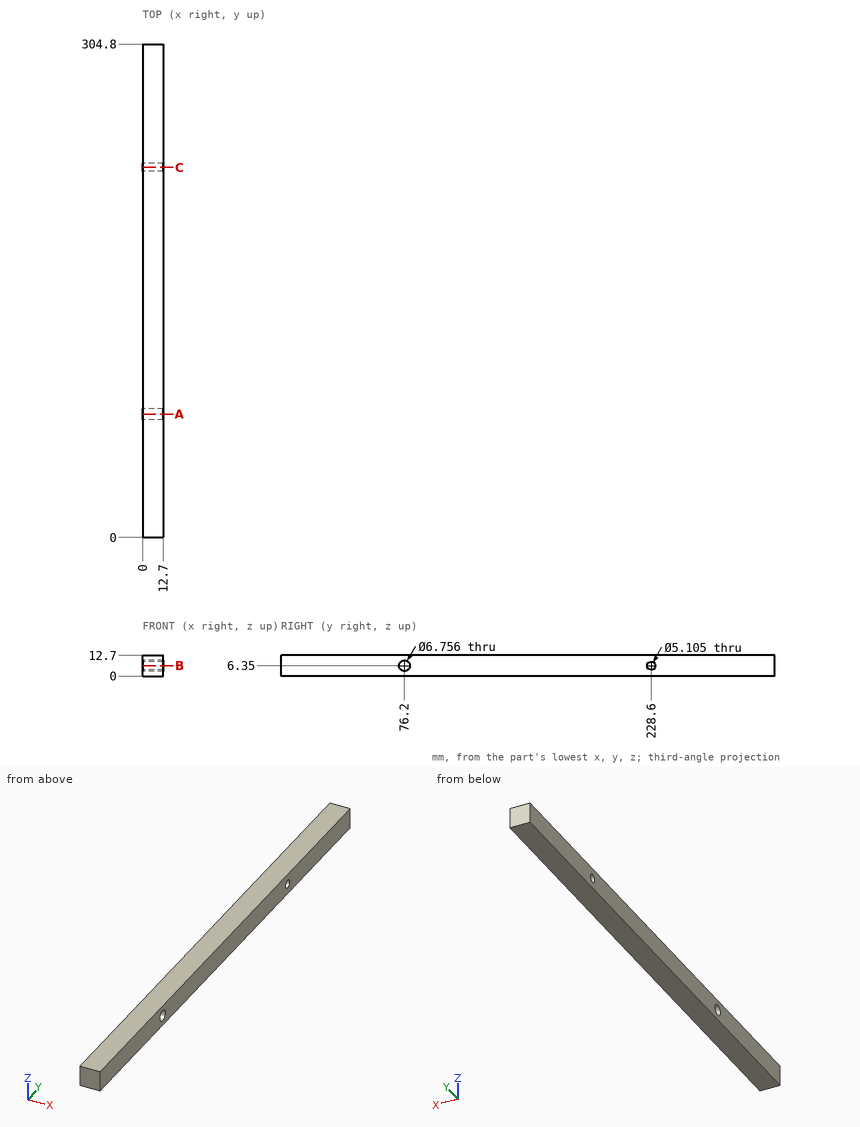
The drawing under review shows one solid part. Ordinate dimensions are in mm from its lowest x, y, z. Round coordinates to 2 decimals unless told otherwise and drop trailing zeros. Loops run counter-clockwise (first coordinate to the right, second up) from the corner with the lowest first, then second, coordinate; pieces in that order, holes last. Notation, with made-up numbers: (-6.75, 53.25) -> (3.25, 53.25) arc R30 cw to (3.25, 77.25) -> close; hole circle Ø7 at (82, 62). An arc over 180 degrees is marked (long way). Answer in a Markdown table with one row per item.
1) Consider section C-C, the plane y = 228.6. Write out the cut boundary in (x, z).
Taken from the geometry:
| item | result |
|---|---|
| outline | (0, 0) -> (12.7, 0) -> (12.7, 3.8) -> (0, 3.8) -> close; (0, 8.9) -> (12.7, 8.9) -> (12.7, 12.7) -> (0, 12.7) -> close |
2) Consider section B-B, the plane z = 6.35. Write out the cut boundary in (x, y), plus the area to 3 significant figures.
Taken from the geometry:
| item | result |
|---|---|
| outline | (0, 0) -> (12.7, 0) -> (12.7, 72.82) -> (0, 72.82) -> close; (0, 79.58) -> (12.7, 79.58) -> (12.7, 226.05) -> (0, 226.05) -> close; (0, 231.15) -> (12.7, 231.15) -> (12.7, 304.8) -> (0, 304.8) -> close |
| area | 3,720 mm² |
3) For pin 1 Ø4 at (y, z) = (228.6, 6.35) entering from +X, flat-tipped, find the tip position at first contact; note if it passes through.
Taken from the geometry:
| item | result |
|---|---|
| pin 1 | passes through |
4) Consider section A-A, the plane y = 76.2. Write out the cut boundary in (x, z).
Taken from the geometry:
| item | result |
|---|---|
| outline | (0, 0) -> (12.7, 0) -> (12.7, 2.97) -> (0, 2.97) -> close; (0, 9.73) -> (12.7, 9.73) -> (12.7, 12.7) -> (0, 12.7) -> close |
5) Wall thickness on line 1 along Z through (x, y) = (6.25, 76.2); line 2 along Z through (x, y) = (9.25, 228.6): over which ranges is each line inside the solid? List them lowest first.
Taken from the geometry:
| item | result |
|---|---|
| line 1 | z = 0 to 2.97, 9.73 to 12.7 |
| line 2 | z = 0 to 3.8, 8.9 to 12.7 |
